Design review of the part built by this model. Coordinates are the model's own, in mm. A direction names the side the tool comes from. Coordinates: 2 decimals unless noted, no trailing zeros. Loops run counter-clockwise (first coordinate to the right, second up) from the corner with the lowest first, then second, coordinate; pieces in that order, holes last. Notation, with made-up numbers: (-12.75, 27) -> (-2.75, 27) arc R9 ccw to (-2.75, 44) -> close; hole circle Ø1 at (-24.5, 79.25). An arc over 180 degrees is marked (long way). Use one line per item in the form item = value. Start each with the question number.
1. Wall thickness on line 1 (Z direction, x = 13, y = 18); line 2 (Y direction, x = 21, z = 5); line 3 (Y direction, x = 16, z = 6): over which ranges is each line inside the solid? List them lowest first. Write a range as from..to.
2. Consider section D-D (y = 28.5). State the section outline as (x, z) points, then the cut area to 3 significant figures.
3. Machinability: for faces 1 (the face through (32, -4, 5)), 2 (the face through (17, 16, 0)), 3 (the face through (3, -4, 5)), which of the approach directions +Z, -Z, +X, -X, +Y, -Y give a long, thin tool a straight path to every point of the face, cutting with its end or side? Answer none if there is none.
4. For pin 1 (17.5 mm diameter, centred on x = 25, y = 22.5, fed in from +Z); pin 2 (1.5 mm diameter, centred on x = 8, z = 5.5, fed in from +Y); pin 3 (4 mm diameter, centred on y = 7, z = 5.5, fed in from +X); pin 4 (5 mm diameter, centred on x = 18.5, z = 5, fed in from +Y), all flat-tipped, find the tip position at first contact; note any pin that passes through.
5. Consider section B-B (y = -1). State the section outline as (x, z) points, then the cut area to 3 significant figures.
6. Consider section C-C (z = 6). State the section outline as (x, y) points.
7. Consider section A-A (x = 30). State the section outline as (y, z) points, then the cut area to 3 significant figures.
from build123d import *

# Parameters (mm, degrees)
F1_W     = 35
F1_H     = 1.6
F4_W     = 3
F4_H     = 8
F5_DEPTH = 5.001


with BuildPart() as f2:
    # F2: sweep along a path in F0
    with BuildLine(Plane.YZ) as f2_path:
        ThreePointArc((-3, 9), (-4.743416, 3.418861), (0, 0))
    # F1 (on Front) → F2 (sweep)
    with BuildSketch(Plane.XZ):
        with Locations((17.5, 0.8)):
            Rectangle(F1_W, F1_H)
    sweep(path=f2_path.line)

    # F3: sweep along a path in F0
    with BuildLine(Plane.YZ) as f3_path:
        Line((0, 0), (32, 0))
    # F1 (on Front) → F3 (sweep)
    with BuildSketch(Plane.XZ):
        with Locations((17.5, 0.8)):
            Rectangle(F1_W, F1_H)
    sweep(path=f3_path.line)

    # F4 (on Front) → F5 (cut, through all)
    with BuildSketch(Plane.XZ):
        with Locations((1.5, 5.6)):
            Rectangle(F4_W, F4_H)
        with Locations((33.5, 5.6)):
            Rectangle(F4_W, F4_H)
    extrude(amount=F5_DEPTH, mode=Mode.SUBTRACT)


solid = f2.part
Geometry check:
q1.line_1 = 0..1.6
q1.line_2 = -5..-3.4
q1.line_3 = -4.9..-3.25
q2.outline = (0, 0) -> (35, 0) -> (35, 1.6) -> (0, 1.6) -> close
q2.area = 56.0 mm²
q3.face_1 = +Z, +X, +Y, -Y
q3.face_2 = -Z, +X, -X, +Y, -Y
q3.face_3 = +Z, -X, +Y, -Y
q4.pin_1 = 1.6
q4.pin_2 = -3.16
q4.pin_3 = through
q4.pin_4 = -2.3
q5.outline = (0, 0.1) -> (35, 0.1) -> (35, 1.6) -> (32, 1.6) -> (32, 1.75) -> (3, 1.75) -> (3, 1.6) -> (0, 1.6) -> close
q5.area = 56.8 mm²
q6.outline = (3, -4.9) -> (32, -4.9) -> (32, -3.25) -> (3, -3.25) -> close
q7.outline = (-3, 9) arc R5 ccw to (0, 0) -> (32, 0) -> (32, 1.6) -> (0, 1.6) arc R3.4 cw to (-2.04, 7.72) -> close
q7.area = 68.0 mm²
